The listing builds one solid part. Answer for the finished solid, in the listing's coordinates (mm). Face numbers are marked on the shaded views. Coordinates: 2 decimals unless noted, no trailing zeros. Loops run counter-clockwise (first coordinate to the right, second up) from the corner with the lowest first, then second, coordinate; pieces in that order, holes last. Notation, with made-up numbers: M 70.5,-11 L 76.5,-11 A25 cw 76.5,2 Z; hole C 57.25,25 d11. An arc over 180 degrees is marked long. Answer as a JSON object with one key per item and string values. Group by question number.
1. A cutting plane is placed at D-D on y = 0. Give the vertices of the cut face in (x, z), and give its area (3 significant figures).
2. Determine the mould class of the marked faces 1, 2 and 3 for opening direction X: released by +X, released by -X, zero draft, split by the parting line, or undercut.
3. A cutting plane is placed at A-A on x = 0. Give the vertices of the cut face in (y, z).
4. A cutting plane is placed at C-C on z = -310. Give the vertices of the cut face in (x, y).
5. Straight lines are drawn through the part: L1, parallel to Y at x = 0, z = 7; L2, parallel to Z at x = 67, y = -239; L3, parallel to X at y = -437, z = -342.5. For each, find the intervals that lie inside material, in ascending order.
6. A cutting plane is placed at B-B on x = -215.9. Give the vertices of the cut face in (y, z).
7. Given pin 1 (16.5 mm diameter, centred on x = -32.004, y = 32.004, fed in from -Z), flat-ended and moving along its own axis, determine where the tip first touches the part or whether it passes through.
from build123d import *

# Parameters (mm, degrees)
F1_DEPTH = 25.4
F2_R     = 25.4
F3_DEPTH = 419.1
F5_D     = 15.875
F7_D     = 12.7


with BuildPart() as f1:
    # F0 (on Top) → F1 (new body)
    with BuildSketch(Plane.XY):
        Polygon((139.7, 215.9), (0, 215.9), (-139.7, 215.9), (-266.7, -469.9), (0, -469.9), (266.7, -469.9), align=None)
    extrude(amount=F1_DEPTH)

    # F2 (on face) → F3 (join)
    with BuildSketch(Plane(origin=(0, 0, 0), x_dir=(1, 0, 0), z_dir=(0, 0, -1))):
        with Locations((-215.9, 419.1)):
            Circle(F2_R)
        with Locations((215.9, 419.1)):
            Circle(F2_R)
        with Locations((0, -165.1)):
            Circle(F2_R)
    extrude(amount=F3_DEPTH)

    # F5 (through all)
    with Locations(Plane.XY.offset(25.4)):
        with Locations((0, 0)):
            Hole(F5_D / 2)

    # F7 (through all)
    with Locations(Plane.XY.offset(25.4)):
        with Locations((32.004, -32.004), (-32.004, -32.004), (32.004, 32.004), (-32.004, 32.004)):
            Hole(F7_D / 2)


solid = f1.part
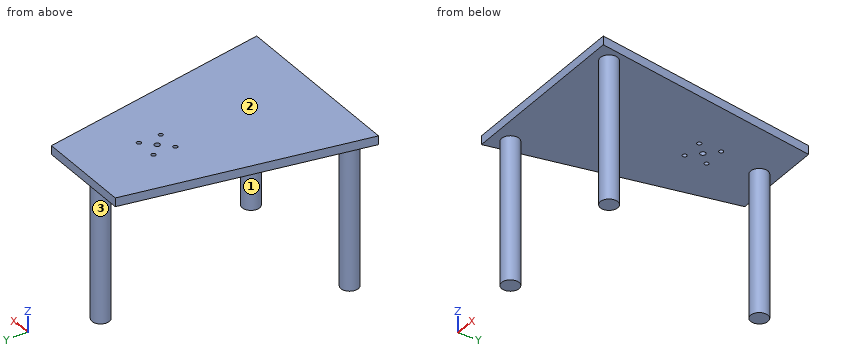
From the geometry:
{
 "1": {"outline": "M -179.68,0 L -7.94,0 L -7.94,25.4 L -179.68,25.4 Z; M 7.94,0 L 179.68,0 L 179.68,25.4 L 7.94,25.4 Z", "area": "8,720 mm²"},
 "2": {"face 1": "undercut", "face 2": "zero draft", "face 3": "split by the parting line"},
 "3": {"outline": "M -469.9,0 L -7.94,0 L -7.94,25.4 L -469.9,25.4 Z; M 7.94,0 L 139.7,0 L 139.7,-419.1 L 190.5,-419.1 L 190.5,0 L 215.9,0 L 215.9,25.4 L 7.94,25.4 Z"},
 "4": {"outline": "C -215.9,-419.1 d50.8; C 0,165.1 d50.8; C 215.9,-419.1 d50.8"},
 "5": {"L1": "y = -469.9 to -7.94, 7.94 to 215.9", "L2": "z = 0 to 25.4", "L3": "x = -233.92 to -197.88, 197.88 to 233.92"},
 "6": {"outline": "M -469.9,0 L -444.5,0 L -444.5,-419.1 L -393.7,-419.1 L -393.7,0 L -195.58,0 L -195.58,25.4 L -469.9,25.4 Z"},
 "7": {"pin 1": "stops at z = 0"}
}
